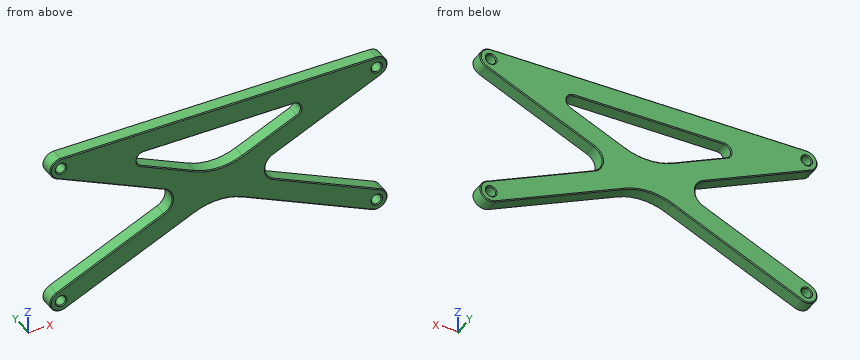
from build123d import *

# Parameters (mm, degrees)
SKETCH1_R           = 2.1828125
BOSS_EXTRUDE1_DEPTH = 6.35
FILLET1_R           = 25.4
FILLET2_R           = 3.175
FILLET3_R           = 6.35
CHAMFER1_SIZE       = 0.396875


with BuildPart() as part:
    # Sketch1 → Boss-Extrude1 (new body)
    with BuildSketch(Plane(origin=(0, 0, 0), x_dir=(1, 0, 0), z_dir=(0, 1, 0))):
        with BuildLine():
            Line((-69.85, -4.7625), (69.85, -4.7625))
            ThreePointArc((69.85, -4.7625), (74.504556808, -1.008219802), (71.820736522, 4.335620349))
            Line((71.820736522, 4.335620349), (11.50910129, 31.75))
            Line((11.50910129, 31.75), (71.820736522, 59.164379651))
            ThreePointArc((71.820736522, 59.164379651), (74.185620349, 65.470736522), (67.879263478, 67.835620349))
            Line((67.879263478, 67.835620349), (0, 36.981409677))
            Line((0, 36.981409677), (-67.879263478, 67.835620349))
            ThreePointArc((-67.879263478, 67.835620349), (-74.185620349, 65.470736522), (-71.820736522, 59.164379651))
            Line((-71.820736522, 59.164379651), (-11.50910129, 31.75))
            Line((-11.50910129, 31.75), (-71.820736522, 4.335620349))
            ThreePointArc((-71.820736522, 4.335620349), (-74.504556808, -1.008219802), (-69.85, -4.7625))
        make_face()
        with Locations((-69.85, 0)):
            Circle(SKETCH1_R, mode=Mode.SUBTRACT)
        with Locations((69.85, 0)):
            Circle(SKETCH1_R, mode=Mode.SUBTRACT)
        with Locations((-69.85, 63.5)):
            Circle(SKETCH1_R, mode=Mode.SUBTRACT)
        with Locations((69.85, 63.5)):
            Circle(SKETCH1_R, mode=Mode.SUBTRACT)
        Polygon((-47.86339871, 4.7625), (47.86339871, 4.7625), (0, 26.518590323), align=None, mode=Mode.SUBTRACT)
    extrude(amount=BOSS_EXTRUDE1_DEPTH)

    # Fillet1
    fillet1_edges = [part.edges().sort_by_distance(p)[0] for p in [
        (0, 3.175, -36.981409677),
        (0, 3.175, -26.518590323),
    ]]
    fillet(fillet1_edges, radius=FILLET1_R)

    # Fillet2
    fillet2_edges = [part.edges().sort_by_distance(p)[0] for p in [
        (47.86339871, 3.175, -4.7625),
        (-47.86339871, 3.175, -4.7625),
    ]]
    fillet(fillet2_edges, radius=FILLET2_R)

    # Fillet3
    fillet3_edges = [part.edges().sort_by_distance(p)[0] for p in [
        (-11.50910129, 3.175, -31.75),
        (11.50910129, 3.175, -31.75),
    ]]
    fillet(fillet3_edges, radius=FILLET3_R)

    # Chamfer1
    chamfer1_edges = [part.edges().sort_by_distance(p)[0] for p in [
        (-48.023828751, 0, -48.347603391),
        (-74.185620349, 0, -65.470736522),
        (39.194929132, 0, -54.797286555),
        (74.504556808, 6.35, 1.008219802),
        (74.185620349, 0, -65.470736522),
        (48.023828751, 0, -15.152396609),
        (74.504556808, 0, 1.008219802),
        (0, 0, 4.7625),
        (-74.504556808, 0, 1.008219802),
        (48.023828751, 6.35, -15.152396609),
        (74.185620349, 6.35, -65.470736522),
        (-72.0328125, 0, 0),
        (-72.0328125, 6.35, 0),
        (39.194929132, 6.35, -54.797286555),
        (67.6671875, 0, 0),
        (67.6671875, 6.35, 0),
        (67.6671875, 0, -63.5),
        (67.6671875, 6.35, -63.5),
        (-74.185620349, 6.35, -65.470736522),
        (-72.0328125, 0, -63.5),
        (-72.0328125, 6.35, -63.5),
        (-48.023828751, 6.35, -48.347603391),
        (-74.504556808, 6.35, 1.008219802),
        (-22.515041825, 0, -16.284480402),
        (-22.515041825, 6.35, -16.284480402),
        (-39.194929132, 0, -54.797286555),
        (-39.194929132, 6.35, -54.797286555),
        (0, 0, -24.017738711),
        (0, 6.35, -24.017738711),
        (0, 0, -39.482261289),
        (0, 6.35, -39.482261289),
        (0, 0, -4.7625),
        (0, 6.35, -4.7625),
        (22.515041825, 6.35, -16.284480402),
        (22.515041825, 0, -16.284480402),
        (36.308702389, 0, -7.265353465),
        (36.308702389, 6.35, -7.265353465),
        (-36.308702389, 0, -7.265353465),
        (-36.308702389, 6.35, -7.265353465),
        (-48.023828751, 0, -15.152396609),
        (-48.023828751, 6.35, -15.152396609),
        (48.023828751, 0, -48.347603391),
        (48.023828751, 6.35, -48.347603391),
        (-20.504569676, 0, -31.75),
        (0, 6.35, 4.7625),
        (-20.504569676, 6.35, -31.75),
        (20.504569676, 0, -31.75),
        (20.504569676, 6.35, -31.75),
    ]]
    chamfer(chamfer1_edges, length=CHAMFER1_SIZE)


solid = part.part
Input: part model. Units: mm. Frame: model coordinates. Coordinates: 2 decimals unless noted, no trailing zeros. Loops run counter-clockwise (first coordinate to the right, second up) from the corner with the lowest first, then second, coordinate; pieces in that order, holes last.
Q1. Contact query for flat-ended pins moving along their axis: pin 1 (5 mm diameter, centred on x = 31, z = -38, fed in from +Y); pin 2 (1.5 mm diameter, centred on y = 5, z = -14, fed in from +X). Output: stop coordinate, or through.
Q2. Material intervals for line 1 (X direction, y = 4.25, z = -1.5); line 2 (X direction, y = 2.2, z = -63.5); line 3 (Z direction, x = -69.85, y = 4.8), sorted ascending.
Q3. Cut plane B-B (y = 4). Give the number of separate pieces and of enclosed holes in the cut face, then the cut area to 3 significant figures.
Q4. Cut plane C-C (x = -55). Output: boundary loops of the cut face in (y, z).
Q5. Cut plane A-A (z = 0). Output: boundary loops of the cut face in (x, y).
Working result:
1. pin 1: stops at y = 6.08
1. pin 2: stops at x = 52.21
2. line 1: x = -74.37 to -71.44, -68.26 to 68.26, 71.44 to 74.37
2. line 2: x = -74.61 to -72.03, -67.67 to -58.34, 58.34 to 67.67, 72.03 to 74.61
2. line 3: z = -68.26 to -65.68, -61.32 to -58.27, -5.23 to -2.18, 2.18 to 4.76
3. separate pieces: 1
3. enclosed holes: 5
3. area: 4,180 mm2
4. outline: (0, -61.55) - (0.4, -61.98) - (5.95, -61.98) - (6.35, -61.55) - (6.35, -51.95) - (5.95, -51.52) - (0.4, -51.52) - (0, -51.95) - close; (0, -11.55) - (0.4, -11.98) - (5.95, -11.98) - (6.35, -11.55) - (6.35, 4.37) - (5.95, 4.76) - (0.4, 4.76) - (0, 4.37) - close
5. outline: (-74.61, 0.4) - (-74.22, 0) - (-72.43, 0) - (-72.03, 0.4) - (-72.03, 5.95) - (-72.43, 6.35) - (-74.22, 6.35) - (-74.61, 5.95) - close; (-67.67, 0.4) - (-67.27, 0) - (67.27, 0) - (67.67, 0.4) - (67.67, 5.95) - (67.27, 6.35) - (-67.27, 6.35) - (-67.67, 5.95) - close; (72.03, 0.4) - (72.43, 0) - (74.22, 0) - (74.61, 0.4) - (74.61, 5.95) - (74.22, 6.35) - (72.43, 6.35) - (72.03, 5.95) - close
